Build history of the part. All positions in model axes, mm. A direction names the side the tool comes from. Give positions to 0.01 mm unless a question says otherwise; leave off trailing zeros. Order: outer loops, then holes, each group sorted by start corner. A loop starts at its lowest first (then second) coordinate and runs counter-clockwise, first axis right, second up. Notation, with made-up numbers: (13.25, 45) - (39.25, 45) arc R16 cw to (39.25, 49) - close; hole circle Ø8 at (35.25, 12.25). An arc over 180 degrees is marked (long way). Use a Markdown table: item, result.
from build123d import *


with BuildPart() as part:
    # Sketch1 → Revolve1 (revolve)
    with BuildSketch(Plane.XY, mode=Mode.PRIVATE) as revolve1_sk:
        Polygon((7.180253608, -6.515318278), (7.180253608, -4.219746392), (5.480253608, -5.919746392), (5.480253608, -8.215318278), align=None)
        Polygon((7.4, -1), (5.480253608, -2.919746392), (5.480253608, -5.919746392), (7.4, -4), align=None)
        Polygon((7.4, -1), (7.4, -4), (11.4, 0), (11.4, 3), (8.4, 0), align=None)
        Polygon((8.4, 0), (11.4, 3), (11.4, 15), (9.9, 15), (9.9, 5), (8.4, 5), align=None)
    revolve(revolve1_sk.sketch.rotate(Axis((0, 51.27419464, 0), (0, -1, 0)), 180), axis=Axis((0, 51.27419464, 0), (0, -1, 0)))


solid = part.part
1) Tool access for faces 1 (the cylindrical face through (2.47, 7.6, 11.13)), 2 (the cylindrical face through (1.6, -5.4, 7)), 3 (the cylindrical face through (-8.012, 2.465, -2.523)): list every direction of +Z, -Z, +X, -X, +Y, -Y with a clear straight run to the whole face (end or side of a thin tool).
Computed:
| item | result |
|---|---|
| face 1 | +Y, -Y |
| face 2 | -Y |
| face 3 | +Y |
2) Pin check, flat tips, straight feed: P1, Ø5, axis at y = 7, z = -5, coming from the +X side; P2, Ø10, axis at x = 8.5, y = -5.5, coming from the -Z side; P3, Ø2, axis at x = -9, z = -1.5, coming from the -Y side; P4, Ø10, axis at x = -2.5, z = 4, coming from the -Y side. Stop position of each tip, or through.
Computed:
| item | result |
|---|---|
| P1 | stops at x = 11.12 |
| P2 | stops at z = -8.29 |
| P3 | stops at y = -3.28 |
| P4 | stops at y = -8.22 |
3) Wall check: line 1 (Z direction, x = 0, y = 2.05); line 2 (Z direction, x = 0, y = 10.25); line 3 (X direction, y = 5.75, z = -3.5). Give the ranges that are in metal, low to high. Write a range as from..to.
Computed:
| item | result |
|---|---|
| line 1 | z = -11.4..-8.4, 8.4..11.4 |
| line 2 | z = -11.4..-9.9, 9.9..11.4 |
| line 3 | x = -10.85..-9.26, 9.26..10.85 |
4) Slice it at C-C (y = -5.5). Write the cut outline in (x, z), and give its area (3 significant figures).
Computed:
| item | result |
|---|---|
| outline | circle Ø14.36 at (0, 0); hole circle Ø10.96 at (0, 0) |
| area | 67.6 mm² |
5) Slice it at D-D (y = 7.25). Write the cut outline in (x, z), and give its area (3 significant figures).
Computed:
| item | result |
|---|---|
| outline | circle Ø22.8 at (0, 0); hole circle Ø19.8 at (0, 0) |
| area | 100 mm² |
6) Slice it at A-A (x = 0). Write the cut outline in (y, z).
Computed:
| item | result |
|---|---|
| outline | (-8.22, -5.48) - (-6.52, -7.18) - (-4.22, -7.18) - (0, -11.4) - (15, -11.4) - (15, -9.9) - (5, -9.9) - (5, -8.4) - (0, -8.4) - (-2.92, -5.48) - close; (-8.22, 5.48) - (-2.92, 5.48) - (0, 8.4) - (5, 8.4) - (5, 9.9) - (15, 9.9) - (15, 11.4) - (0, 11.4) - (-4.22, 7.18) - (-6.52, 7.18) - close |
7) Slice it at B-B (z = 0). Write the cut outline in (x, y).
Computed:
| item | result |
|---|---|
| outline | (-11.4, 0) - (-7.18, -4.22) - (-7.18, -6.52) - (-5.48, -8.22) - (-5.48, -2.92) - (-8.4, 0) - (-8.4, 5) - (-9.9, 5) - (-9.9, 15) - (-11.4, 15) - close; (5.48, -8.22) - (7.18, -6.52) - (7.18, -4.22) - (11.4, 0) - (11.4, 15) - (9.9, 15) - (9.9, 5) - (8.4, 5) - (8.4, 0) - (5.48, -2.92) - close |
8) Two-plate mould, pull along Z, no slides. Class faces 4 (the flat face through (2.98, 5, 8.02)), 5 (the conical face through (-7.1, -3.956, -2.236)), 6 (the flat face through (0.1, 15, -10.2)), 7 (the cylindrical face through (-9.443, 9.93, -2.974)): +Z half, -Z half, draft (parallel to the pull), parting line (faces both ways), or undercut.
Computed:
| item | result |
|---|---|
| face 4 | undercut |
| face 5 | parting line |
| face 6 | draft |
| face 7 | undercut |
